```python
from build123d import *

# Parameters (mm, degrees)
SKETCH1_W           = 242
SKETCH1_H           = 350
SKETCH1_R           = 13
BOSS_EXTRUDE1_DEPTH = 10
SKETCH2_W           = 40
SKETCH2_H           = 350
CUT_EXTRUDE1_DEPTH  = 0.5
SKETCH3_W           = 10
SKETCH3_H           = 100
CUT_EXTRUDE2_DEPTH  = 11
FILLET1_R           = 10


with BuildPart() as part:
    # Sketch1 → Boss-Extrude1 (new body)
    with BuildSketch(Plane.XY):
        Rectangle(SKETCH1_W, SKETCH1_H)
        with Locations((-103, 140)):
            Circle(SKETCH1_R, mode=Mode.SUBTRACT)
        with Locations((-103, -140)):
            Circle(SKETCH1_R, mode=Mode.SUBTRACT)
        with Locations((103, 140)):
            Circle(SKETCH1_R, mode=Mode.SUBTRACT)
        with Locations((103, -140)):
            Circle(SKETCH1_R, mode=Mode.SUBTRACT)
    extrude(amount=BOSS_EXTRUDE1_DEPTH)

    # Sketch2 → Cut-Extrude1 (cut)
    with BuildSketch(Plane.XY.offset(10)):
        with Locations((-101, 0)):
            Rectangle(SKETCH2_W, SKETCH2_H)
        with Locations((101, 0)):
            Rectangle(SKETCH2_W, SKETCH2_H)
    extrude(amount=-CUT_EXTRUDE1_DEPTH, mode=Mode.SUBTRACT)

    # Sketch3 → Cut-Extrude2 (cut, through all)
    with BuildSketch(Plane.XY.offset(10)):
        with Locations((0, 125)):
            Rectangle(SKETCH3_W, SKETCH3_H)
    extrude(amount=-CUT_EXTRUDE2_DEPTH, mode=Mode.SUBTRACT)

    # Fillet1
    fillet1_edges = [part.edges().sort_by_distance(p)[0] for p in [
        (5, 175, 5),
        (-5, 175, 5),
    ]]
    fillet(fillet1_edges, radius=FILLET1_R)


solid = part.part
```
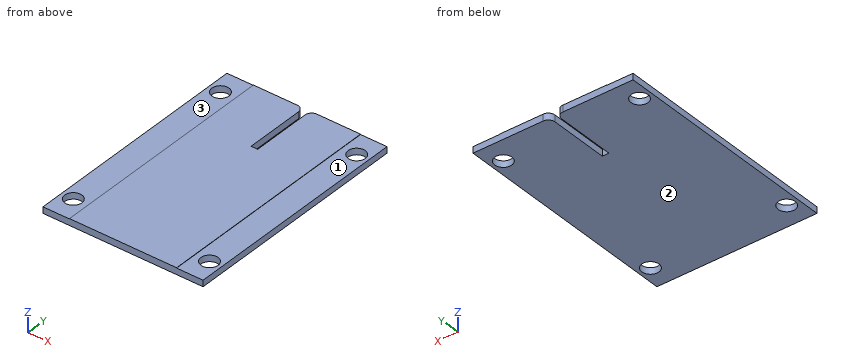
The model under review builds one solid part; all positions refer to its coordinate system, in mm. Face numbers are marked on the shaded views. A direction names the side the tool comes from. Round coordinates to 2 decimals unless told otherwise and drop trailing zeros. Order: outer loops, then holes, each group sorted by start corner. A loop starts at its lowest first (then second) coordinate and runs counter-clockwise, first axis right, second up. Notation, with made-up numbers: M 69.5,76 L 99.5,76 A21 cw 99.5,110 Z; hole C -10,38 d10. An arc over 180 degrees is marked long. Use a Markdown table: item, result.
1) Insertion check: pin 1 (21 mm diameter, centred on x = 103, y = 140, fed in from +Z). The pin has a flat end and moves straight along its axis. Give the tip position at first contact, or say it passes through.
Report:
| item | result |
|---|---|
| pin 1 | through |
2) Consider section D-D (y = 140). Write out the cut boundary in (x, z).
Report:
| item | result |
|---|---|
| outline | M -121,0 L -116,0 L -116,9.5 L -121,9.5 Z; M -90,0 L -5,0 L -5,10 L -81,10 L -81,9.5 L -90,9.5 Z; M 5,0 L 90,0 L 90,9.5 L 81,9.5 L 81,10 L 5,10 Z; M 116,0 L 121,0 L 121,9.5 L 116,9.5 Z |
3) Consider section B-B (z = 7). Write out the cut boundary in (x, y), then the cut area to 3 significant figures.
Report:
| item | result |
|---|---|
| outline | M -121,-175 L 121,-175 L 121,175 L 15,175 A10 ccw 5,165 L 5,75 L -5,75 L -5,165 A10 ccw -15,175 L -121,175 Z; hole C -103,-140 d26; hole C -103,140 d26; hole C 103,-140 d26; hole C 103,140 d26 |
| area | 81,500 mm^2 |
4) Tool access review of the marked faces 1, 2 and 3: name each direction out of +Z, -Z, +X, -X, +Y, -Y from which nothing blocks a thin tool from reaching the whole face with its end or side.
Report:
| item | result |
|---|---|
| face 1 | +Z, +X, +Y, -Y |
| face 2 | -Z, +X, -X, +Y, -Y |
| face 3 | +Z, -X, +Y, -Y |
5) Wall thickness on line 1 along X through (y, z) = (-140, 5); line 2 along Y through (x, z) = (103, 5.5); line 3 along X through (y, z) = (140, 6.25): over which ranges is each line inside the solid? List them lowest first. Write a range as [from, to].
Report:
| item | result |
|---|---|
| line 1 | [-121, -116], [-90, 90], [116, 121] |
| line 2 | [-175, -153], [-127, 127], [153, 175] |
| line 3 | [-121, -116], [-90, -5], [5, 90], [116, 121] |
6) Consider section C-C (x = -103). Write out the cut boundary in (y, z).
Report:
| item | result |
|---|---|
| outline | M -175,0 L -153,0 L -153,9.5 L -175,9.5 Z; M -127,0 L 127,0 L 127,9.5 L -127,9.5 Z; M 153,0 L 175,0 L 175,9.5 L 153,9.5 Z |
7) Consider section A-A (y = -140). Write out the cut boundary in (x, z).
Report:
| item | result |
|---|---|
| outline | M -121,0 L -116,0 L -116,9.5 L -121,9.5 Z; M -90,0 L 90,0 L 90,9.5 L 81,9.5 L 81,10 L -81,10 L -81,9.5 L -90,9.5 Z; M 116,0 L 121,0 L 121,9.5 L 116,9.5 Z |
